```python
from build123d import *

# Parameters (mm, degrees)
SKETCH_1_W          = 7
SKETCH_1_H          = 60
SKETCH_1_W_2        = 75
SKETCH_1_H_2        = 7
EXTRUDE_1_DEPTH     = 35
EXTRUDE_2_DEPTH     = 6
SKETCH_3_W          = 45
SKETCH_3_H          = 8
CUT_EXTRUDE_1_DEPTH = 3
SKETCH_4_W          = 15
SKETCH_4_H          = 12
CUT_EXTRUDE_2_DEPTH = 106.858395983
CUT_EXTRUDE_3_DEPTH = 2


with BuildPart() as part:
    # Эскиз1 → Бобышка-Вытянуть1 (new body)
    with BuildSketch(Plane.XY):
        with Locations((3.5, 37)):
            Rectangle(SKETCH_1_W, SKETCH_1_H)
        with Locations((37.5, 3.5)):
            Rectangle(SKETCH_1_W_2, SKETCH_1_H_2)
    extrude_1 = extrude(amount=EXTRUDE_1_DEPTH)

    # Эскиз2 → Бобышка-Вытянуть2 (add)
    with BuildSketch(Plane(origin=(0, 67, 0), x_dir=(1, 0, 0), z_dir=(0, 1, 0))):
        Polygon((0, -35), (65, -35), (65, -17), (7, 0), (0, 0), align=None)
    extrude_2 = extrude(amount=EXTRUDE_2_DEPTH)

    # Эскиз3 → Вырез-Вытянуть1 (cut)
    with BuildSketch(Plane(origin=(0, 73, 0), x_dir=(1, 0, 0), z_dir=(0, 1, 0))):
        with Locations((22.5, -31)):
            Rectangle(SKETCH_3_W, SKETCH_3_H)
    cut_extrude_1 = extrude(amount=-CUT_EXTRUDE_1_DEPTH, mode=Mode.SUBTRACT)

    # Эскиз4 → Вырез-Вытянуть2 (cut, through all)
    with BuildSketch(Plane(origin=(0, 7, 0), x_dir=(1, 0, 0), z_dir=(0, 1, 0))):
        with Locations((47.5, -6)):
            Rectangle(SKETCH_4_W, SKETCH_4_H)
    cut_extrude_2 = extrude(amount=-CUT_EXTRUDE_2_DEPTH, mode=Mode.SUBTRACT)

    # Зеркальное отражение1: Бобышка-Вытянуть1, Бобышка-Вытянуть2, Вырез-Вытянуть1, Вырез-Вытянуть2 across plane
    add(extrude_1.mirror(Plane.XY.offset(35)))
    add(extrude_2.mirror(Plane.XY.offset(35)))
    add(cut_extrude_1.mirror(Plane.XY.offset(35)), mode=Mode.SUBTRACT)
    add(cut_extrude_2.mirror(Plane.XY.offset(35)), mode=Mode.SUBTRACT)

    # Эскиз5 → Вырез-Вытянуть3 (cut)
    with BuildSketch(Plane.ZY):
        Polygon((70, 73), (43, 73), (43, 70), (27, 70), (27, 73), (0, 73), (0, 0), (70, 0), align=None)
    extrude(amount=-CUT_EXTRUDE_3_DEPTH, mode=Mode.SUBTRACT)


solid = part.part
```
Can you work these out from the model? Positions are in its coordinate system, mm. A direction names the side the tool comes from. Coordinates: 2 decimals unless noted, no trailing zeros. Loops run counter-clockwise (first coordinate to the right, second up) from the corner with the lowest first, then second, coordinate; pieces in that order, holes last.
1) Which directions (+Z, -Z, +X, -X, +Y, -Y) give clear straight access to the entire face, cutting with the end or side of a thin tool? Please do faces 4 (the flat face through (47, 4, 12)), 5 (the flat face through (23, 72, 43)), 6 (the flat face through (41, 7, 35)).
2) Imagine slicing it at B-B on z = 36. List the corners of the cut face in (x, y) for me.
3) Imagine slicing it at C-C on x = 41. List the corners of the cut face in (y, z) for me.
4) For pin 1 (5 mm diameter, centred on x = 19, z = 32, fed in from +Y); pin 2 (3.5 mm diameter, centred on x = 50, y = 3.5, fed in from +Z); pin 3 (1.5 mm diameter, centred on x = 17.5, y = 71.5, fed in from -Z), each with a flat end and sliding along its axis, tell me the tip position at first contact or that it passes through.
5) Imagine slicing it at D-D on y = 26. List the corners of the cut face in (x, z) for me.
6) I need wall thicknesses on probe 1 along Y at (x, z) = (16, 62); probe 2 along X at (y, z) = (41, 29); probe 3 along Y at (x, z) = (34, 6). Which ranges of each line are inside material? Lowest first, please.
7) Imagine slicing it at A-A on x = 50.5. List the corners of the cut face in (y, z) for me.
8) Thinking about a two-plate mould opening in Y: for faces 1 (the flat face through (38, 0, 35)), 2 (the flat face through (36.41, 69.96, 8.62)), 3 (the flat face through (29, 67, 35)), which applies, pulls with the +Y half, pulls with the -Y half, needs draft (parallel to the pull), parting line crosses it, or undercut?
Completed:
1. face 4: -Z, -Y
1. face 5: -X, +Y
1. face 6: +Z, -Z, +X
2. outline: (2, 0) - (75, 0) - (75, 7) - (7, 7) - (7, 67) - (65, 67) - (65, 73) - (45, 73) - (45, 70) - (2, 70) - close
3. outline: (0, 12) - (7, 12) - (7, 58) - (0, 58) - close; (67, 9.97) - (73, 9.97) - (73, 27) - (70, 27) - (70, 43) - (73, 43) - (73, 60.03) - (67, 60.03) - close
4. pin 1: stops at y = 70
4. pin 2: stops at z = 58
4. pin 3: stops at z = 2.86
5. outline: (2, 0) - (7, 0) - (7, 70) - (2, 70) - close
6. probe 1: y = 0 to 7, 67 to 73
6. probe 2: x = 2 to 7
6. probe 3: y = 0 to 7
7. outline: (0, 12) - (7, 12) - (7, 58) - (0, 58) - close; (67, 12.75) - (73, 12.75) - (73, 57.25) - (67, 57.25) - close
8. face 1: pulls with the -Y half
8. face 2: needs draft
8. face 3: undercut
